The model under review builds one solid part; all positions refer to its coordinate system, in mm. Coordinates: 2 decimals unless noted, no trailing zeros. Order: outer loops, then holes, each group sorted by start corner. A loop starts at its lowest first (then second) coordinate and runs counter-clockwise, first axis right, second up. Notation, with made-up numbers: (61.25, 38.5) -> (96.25, 38.5) arc R23 ccw to (96.25, 73.5) -> close; hole circle Ø7 at (-22, 46.5). An arc over 180 degrees is marked (long way). Put each result on its own line as item: value.
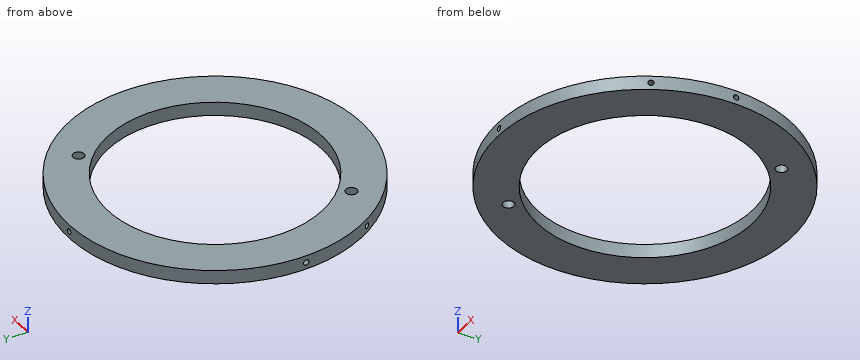
from build123d import *

# Parameters (mm, degrees)
SKETCH1_R         = 68.1355
SKETCH1_R_2       = 49.8475
EXTRUDE1_DEPTH    = 6.35
CIRPATTERN1_COUNT = 4
CIRPATTERN3_COUNT = 3
CIRPATTERN2_COUNT = 2


with BuildPart() as part:
    # Sketch1 → Extrude1 (new body)
    with BuildSketch(Plane.XY):
        Circle(SKETCH1_R)
        Circle(SKETCH1_R_2, mode=Mode.SUBTRACT)
    extrude(amount=EXTRUDE1_DEPTH)

    # Sketch4 → M3x0.5 Tapped Hole1 (revolve, cut)
    with BuildSketch(Plane(origin=(0, 68.1355, 3.175), x_dir=(0, 0, 1), z_dir=(1, 0, 0))):
        Polygon((0, 0), (0, 9.387075774), (1.25, 8.636), (1.25, 0), align=None)
    m3x0_5_tapped_hole1 = revolve(axis=Axis((0, 74.4855, 3.175), (0, -1, 0)), mode=Mode.SUBTRACT)

    # CirPattern1: M3x0.5 Tapped Hole1 ×4 about axis
    cirpattern1_axis = Axis((0, 0, 6.35), (0, 0, -1))
    for i in range(1, CIRPATTERN1_COUNT):
        add(m3x0_5_tapped_hole1.rotate(cirpattern1_axis, i * 360 / CIRPATTERN1_COUNT), mode=Mode.SUBTRACT)

    # CirPattern3: M3x0.5 Tapped Hole1 ×3 about axis
    cirpattern3_axis = Axis((0, 0, 6.35), (0, 0, -1))
    for i in range(1, CIRPATTERN3_COUNT):
        add(m3x0_5_tapped_hole1.rotate(cirpattern3_axis, i * 360 / CIRPATTERN3_COUNT), mode=Mode.SUBTRACT)

    # Sketch18 → 1/4-20 Tapped Hole1 (revolve, cut)
    with BuildSketch(Plane(origin=(39.207798225, 39.207798225, 6.35), x_dir=(0, -1, 0), z_dir=(1, 0, 0))):
        Polygon((0, 0), (0, 20.583816902), (2.5527, 19.05), (2.5527, 0), align=None)
    f_1_4_20_tapped_hole1 = revolve(axis=Axis((39.207798225, 39.207798225, 12.7), (0, 0, -1)), mode=Mode.SUBTRACT)

    # CirPattern2: 1/4-20 Tapped Hole1 ×2 about axis
    cirpattern2_axis = Axis((0, 0, 0), (0, 0, 1))
    for i in range(1, CIRPATTERN2_COUNT):
        add(f_1_4_20_tapped_hole1.rotate(cirpattern2_axis, i * 360 / CIRPATTERN2_COUNT), mode=Mode.SUBTRACT)


solid = part.part
Item 1: For pin 1 Ø3 at (x, z) = (-38.5, 1.5) entering from +Y; pin 2 Ø1.5 at (y, z) = (-33, 4) entering from -X; pin 3 Ø1.5 at (y, z) = (0, 3.175) entering from -X, all flat-tipped, find the tip position at first contact; note any pin that passes through.
Answers below:
pin 1: y = 57.21
pin 2: x = -60.02
pin 3: x = -59.2
Item 2: Consider section B-B on x = -34.5. Write out the cut boundary in (y, z), and give its area (3 significant figures).
Answers below:
outline: (-58.76, 0) -> (-35.98, 0) -> (-35.98, 6.35) -> (-58.76, 6.35) -> close; (35.98, 0) -> (58.76, 0) -> (58.76, 6.35) -> (35.98, 6.35) -> close
area: 289 mm^2
Item 3: Consider section C-C on y = -56.5. Write out the cut boundary in (x, z), and give its area (3 significant figures).
Answers below:
outline: (-38.08, 0) -> (38.08, 0) -> (38.08, 6.35) -> (-38.08, 6.35) -> close
area: 484 mm^2
Item 4: Consider section A-A on y = 45. Write out the cut boundary in (x, z).
Answers below:
outline: (-51.16, 0) -> (-21.44, 0) -> (-21.44, 6.35) -> (-51.16, 6.35) -> close; (21.44, 0) -> (51.16, 0) -> (51.16, 6.35) -> (21.44, 6.35) -> close
Item 5: For line 1 (Y direction, x = -37.5, z = 1); line 2 (Z direction, x = 0, y = 62.25) (3 decimals); line 3 (X direction, y = -39, z = 4.75), list the stretches that pass through material, from the lowest coordinate up. Write a range as from..to.
Answers below:
line 1: -56.89..-41.11, -37.31..-32.84, 32.84..56.89
line 2: 0..1.925, 4.425..6.35
line 3: -55.87..-41.75, -36.66..-31.04, 31.04..55.87
